from build123d import *

# Parameters (mm, degrees)
SKETCH1_R           = 2.6
BOSS_EXTRUDE3_DEPTH = 10
SKETCH5_R           = 5
CUT_EXTRUDE3_DEPTH  = 20
FILLET2_R           = 1


with BuildPart() as part:
    # Sketch1 → Boss-Extrude3 (new body)
    with BuildSketch(Plane(origin=(0, 0, 0), x_dir=(1, 0, 0), z_dir=(0, 1, 0))):
        with BuildLine():
            Line((-13.5, -10), (13.5, -10))
            ThreePointArc((13.5, -10), (15.621320344, -9.121320344), (16.5, -7))
            Line((16.5, -7), (16.5, 7))
            ThreePointArc((16.5, 7), (15.621320344, 9.121320344), (13.5, 10))
            Line((13.5, 10), (-13.5, 10))
            ThreePointArc((-13.5, 10), (-15.621320344, 9.121320344), (-16.5, 7))
            Line((-16.5, 7), (-16.5, -7))
            ThreePointArc((-16.5, -7), (-15.621320344, -9.121320344), (-13.5, -10))
        make_face()
        with Locations(Location((10.5, 0, 0), (0, 0, 270))):
            Circle(SKETCH1_R, mode=Mode.SUBTRACT)
        with Locations(Location((-10.5, 0, 0), (0, 0, 90))):
            Circle(SKETCH1_R, mode=Mode.SUBTRACT)
    extrude(amount=BOSS_EXTRUDE3_DEPTH)

    # Sketch5 → Cut-Extrude3 (cut)
    with BuildSketch(Plane(origin=(0, 0, -10), x_dir=(-1, 0, 0), z_dir=(0, 0, -1))):
        with Locations((0, 10.1)):
            Circle(SKETCH5_R)
    extrude(amount=-CUT_EXTRUDE3_DEPTH, mode=Mode.SUBTRACT)

    # Fillet2
    fillet2_edges = [part.edges().sort_by_distance(p)[0] for p in [
        (0, 0, 10),
        (-15.621320344, 0, 9.121320344),
        (-16.5, 0, 0),
        (-15.621320344, 0, -9.121320344),
        (0, 0, -10),
        (15.621320344, 0, -9.121320344),
        (16.5, 0, 0),
        (15.621320344, 0, 9.121320344),
    ]]
    fillet(fillet2_edges, radius=FILLET2_R)


solid = part.part
Part model, mm, in its own coordinate system. Give positions to 0.01 mm unless a question says otherwise; leave off trailing zeros. Loops run counter-clockwise (first coordinate to the right, second up) from the corner with the lowest first, then second, coordinate; pieces in that order, holes last. Notation, with made-up numbers: (22.25, 0.25) -> (56.25, 0.25) arc R27 ccw to (56.25, 38.25) -> close; hole circle Ø7 at (55.25, 44.25). An arc over 180 degrees is marked (long way). Write each question's results on one line, items separated by ' | '. Start each with the question number.
Q1. Band-saw the part on B-B on y = 2.25. List the corners of the cut face in (x, z).
Q2. Pin check, flat tip, straight feed: P1, Ø4.5, axis at x = 10.5, z = 0, coming from the +Y side. Stop position of the tip, or through.
Q3. Band-saw the part on D-D on y = 9.25. List the corners of the cut face in (x, z).
Q4. Band-saw the part on C-C on x = 10.5. List the corners of the cut face in (y, z).
Q5. Band-saw the part on A-A on z = 0. List the corners of the cut face in (x, y).
Q6. Pull direction X, two halves, no side cores. Call faces 1 (the face through (-15.64, 5.44, 9.1)), 2 (the face through (7.96, 4.93, -0.56)), 3 (the face through (0, 4, -10)): +X half, -X half, draft (parallel to the pull), parting line (faces both ways), or undercut.
Q7. Wall check: L1, parallel to X at y = 2.5, z = 0; L2, parallel to Z at x = -10.5, y = 4.75; L3, parallel to X at y = 3.5, z = 2. Give the ranges that are in metal, low to high.
Results are:
1) outline: (-16.5, -7) arc R3 ccw to (-13.5, -10) -> (13.5, -10) arc R3 ccw to (16.5, -7) -> (16.5, 7) arc R3 ccw to (13.5, 10) -> (-13.5, 10) arc R3 ccw to (-16.5, 7) -> close; hole circle Ø5.2 at (-10.5, 0); hole circle Ø5.2 at (10.5, 0)
2) P1: passes through
3) outline: (-16.5, -7) arc R3 ccw to (-13.5, -10) -> (-4.93, -10) -> (-4.93, 10) -> (-13.5, 10) arc R3 ccw to (-16.5, 7) -> close; (4.93, -10) -> (13.5, -10) arc R3 ccw to (16.5, -7) -> (16.5, 7) arc R3 ccw to (13.5, 10) -> (4.93, 10) -> close; hole circle Ø5.2 at (-10.5, 0); hole circle Ø5.2 at (10.5, 0)
4) outline: (0, -9) arc R1 ccw to (1, -10) -> (10, -10) -> (10, -2.6) -> (0, -2.6) -> close; (0, 2.6) -> (10, 2.6) -> (10, 10) -> (1, 10) arc R1 ccw to (0, 9) -> close
5) outline: (-16.5, 1) arc R1 ccw to (-15.5, 0) -> (-13.1, 0) -> (-13.1, 10) -> (-16.5, 10) -> close; (-7.9, 0) -> (7.9, 0) -> (7.9, 10) -> (5, 10) arc R5 cw to (-5, 10) -> (-7.9, 10) -> close; (13.1, 0) -> (15.5, 0) arc R1 ccw to (16.5, 1) -> (16.5, 10) -> (13.1, 10) -> close
6) face 1: -X half | face 2: undercut | face 3: draft
7) L1: x = -16.5 to -13.1, -7.9 to 7.9, 13.1 to 16.5 | L2: z = -10 to -2.6, 2.6 to 10 | L3: x = -16.5 to -12.16, -8.84 to 8.84, 12.16 to 16.5
